from build123d import *

# Parameters (mm, degrees)
SKETCH1_W           = 20
SKETCH1_H           = 49.25
BOSS_EXTRUDE1_DEPTH = 2.5
FILLET3_R           = 2.5
CUT_EXTRUDE1_START  = -16
CUT_EXTRUDE1_DEPTH  = 35.317119353
SKETCH14_R          = 2
BOSS_EXTRUDE2_DEPTH = 5.5


with BuildPart() as part:
    # Sketch1 → Boss-Extrude1 (new, symmetric)
    with BuildSketch(Plane.XY):
        with Locations((0, 24.625)):
            Rectangle(SKETCH1_W, SKETCH1_H)
    extrude(amount=BOSS_EXTRUDE1_DEPTH, both=True)

    # Fillet3
    fillet3_edges = [part.edges().sort_by_distance(p)[0] for p in [
        (10, 24.625, 2.5),
        (10, 24.625, -2.5),
    ]]
    fillet(fillet3_edges, radius=FILLET3_R - 0.0001)  # a hair under: the kernel refuses the full size

    # Sketch11 → Cut-Extrude1 (cut, through all)
    with BuildSketch(Plane(origin=(0, 49.25, 0), x_dir=(1, 0, 0), z_dir=(0, 1, 0)).offset(CUT_EXTRUDE1_START)):
        Polygon((-10, 1), (7.5, 2.5), (-10, 2.5), align=None)
        Polygon((7.5, -2.5), (-10, -1), (-10, -2.5), align=None)
    extrude(amount=-CUT_EXTRUDE1_DEPTH, mode=Mode.SUBTRACT)

    # Sketch14 → Boss-Extrude2 (add, symmetric)
    with BuildSketch(Plane.XY):
        with Locations((0, 39.25)):
            Circle(SKETCH14_R)
    extrude(amount=BOSS_EXTRUDE2_DEPTH, both=True)


solid = part.part
Work out the finished part from the listing and answer in its coordinate system (mm). A direction names the side the tool comes from. Coordinates: 2 decimals unless noted, no trailing zeros. Write each loop counter-clockwise with the first axis right and the second up, starting at its lowest first coordinate (ties: lowest second). Pieces come first, ordered by that corner, then holes.
1. For faces 1 (the flat face through (-5, 33.25, 2)), 2 (the cylindrical face through (-0.434, 37.298, -3.979)), 3 (the cylindrical face through (9, 25, -2)), 4 (the flat face through (-3, 33.25, -2)), determine the directions among +Z, -Z, +X, -X, +Y, -Y from which every point of the face is accessible in a straight line to the end or side of a thin tool.
Results list:
face 1: +Z, -X, -Y
face 2: -Z
face 3: -Z, +X, +Y, -Y
face 4: -Z, -X, -Y
2. The part is cut by section C-C, the plane z = 4.25. Write down the section's boundary in (x, y).
Results list:
outline: circle Ø4 at (0, 39.25)
3. Consider line 1 along Z through (x, y) = (-5.25, 37.5); line 2 along Y through (x, z) = (-6.75, 1.75); line 3 along Z through (x, y) = (-4, 6). Determine where each line is inside the solid, lowest interval first.
Results list:
line 1: z = -2.5 to 2.5
line 2: y = 33.25 to 49.25
line 3: z = -1.51 to 1.51
4. For a pull along Y with two mould halves and no side action, classify faces 5 (the flat face through (2, 0, 0)), 6 (the cylindrical face through (9, 25, 2)), 7 (the cylindrical face through (-0.434, 37.298, 4.021)) as +Y half, -Y half, draft (parallel to the pull), parting line (faces both ways), or undercut.
Results list:
face 5: -Y half
face 6: draft
face 7: parting line
5. Flat-ended cylindrical pins translate along their axes: pin 1 (4 mm diameter, centred on y = 15.5, z = -3, fed in from +X); pin 2 (1.5 mm diameter, centred on x = 1, z = 4, fed in from -Y); pin 3 (5.5 mm diameter, centred on x = -3.5, y = 15.5, fed in from -Z). Find the tip coordinate at first contact, or state that the pin passes through.
Results list:
pin 1: stops at x = 9.79
pin 2: stops at y = 37.27
pin 3: stops at z = -1.79
6. The part is cut by section A-A, the plane x = 4. Write down the section's boundary in (y, z).
Results list:
outline: (0, -2.2) - (33.25, -2.2) - (33.25, -2.5) - (49.25, -2.5) - (49.25, 2.5) - (33.25, 2.5) - (33.25, 2.2) - (0, 2.2) - close
